Here's how the part is built. I have some questions about the finished solid (model axes, mm). A direction names the side the tool comes from. Give positions to 0.01 mm unless a question says otherwise; leave off trailing zeros. Loops run counter-clockwise (first coordinate to the right, second up) from the corner with the lowest first, then second, coordinate; pieces in that order, holes last. Notation, with made-up numbers: M 34.25,49 L 93.25,49 A25 cw 93.25,84 Z; hole C 56.25,0.5 d3. An arc over 180 degrees is marked long. Write item = value, one per line. Start each with the question number.
```python
from build123d import *

# Parameters (mm, degrees)
SKETCH_1_R      = 41.5
EXTRUDE_1_DEPTH = 2


with BuildPart() as part:
    # 草图1 → 凸台-拉伸1 (new body)
    with BuildSketch(Plane.XY):
        with BuildLine():
            Line((3, -140.066053532), (3, -45.918827896))
            ThreePointArc((3, -45.918827896), (31.460201745, 33.582651198), (-46.016722562, 0))
            Line((-46.016722562, 0), (-46.016722562, -112.361648418))
            ThreePointArc((-46.016722562, -112.361648418), (-37.365245186, -155.855562297), (-12.727922061, -192.727922061))
            ThreePointArc((-12.727922061, -192.727922061), (12.295990665, -193.145669004), (13.548765941, -168.149643825))
            ThreePointArc((13.548765941, -168.149643825), (5.724176996, -155.065757751), (3, -140.066053532))
        make_face()
        Circle(SKETCH_1_R, mode=Mode.SUBTRACT)
    extrude(amount=EXTRUDE_1_DEPTH)


solid = part.part
```
Q1. Will these pins go through, and if not, where does the flat tip stop? pin 1 (1 mm diameter, centred on y = -106, z = 1, fed in from +X); pin 2 (1 mm diameter, centred on x = 26, z = 1, fed in from +Y).
Q2. If we section it at B-B, the plane x = 0: List the corners of the cut face in (y, z) for me.
Q3. If we section it at D-D, the plane x = -10.5: List the corners of the cut face in (y, z) for me, then the cut area to 3 significant figures.
Q4. If we section it at C-C, the plane y = -104: List the corners of the cut face in (x, z) for me, then the cut area to 3 significant figures.
Q5. If I drill on line 1 along Y through (x, z) = (0, 1.55); line 2 along Y through (x, z) = (12, 0.45); line 3 along X through (y, z) = (-14, 1.85), over which ranges is the centre line in solid material (lowest first)?
Q6. We'd pull the mould along X, two halves only. Please class faces 3 (the cylindrical face through (39.584, 12.465, 0.986)), 4 (the cylindrical face through (-37.6, -155.28, 0.99)), 5 (the cylindrical face through (32.54, 32.54, 0.99)), 6 (the flat face through (-21, -101, 2)): pulls with the +X half, pulls with the -X half, needs draft (parallel to the pull), parting line crosses it, or undercut.
Q7. If we section it at A-A, the plane z = 1.45: List the corners of the cut face in (x, y) for me, then the cut area to 3 significant figures.
Q8. On a 3-axis mill with a long thin cutter (end or side, diameter ignored), from which of +Z, -Z, +X, -X, +Y, -Y can I reach the whole of each face in a straight line? I mean faces 1 (the cylindrical face through (12.01, -193.41, 0.99)), 2 (the cylindrical face through (5.8, -155.27, 0.99)). Say none if no direction works.
Resolved:
q1.pin_1 = 3
q1.pin_2 = 38.31
q2.outline = M -198,0 L -41.5,0 L -41.5,2 L -198,2 Z; M 41.5,0 L 46.02,0 L 46.02,2 L 41.5,2 Z
q3.outline = M -194.62,0 L -40.15,0 L -40.15,2 L -194.62,2 Z; M 40.15,0 L 44.8,0 L 44.8,2 L 40.15,2 Z
q3.area = 318 mm²
q4.outline = M -46.02,0 L 3,0 L 3,2 L -46.02,2 Z
q4.area = 98.0 mm²
q5.line_1 = -198 to -41.5, 41.5 to 46.02
q5.line_2 = -193.42 to -166.27, -44.42 to -39.73, 39.73 to 44.42
q5.line_3 = -46.02 to -39.07, 39.07 to 43.84
q6.face_3 = undercut
q6.face_4 = pulls with the -X half
q6.face_5 = parting line crosses it
q6.face_6 = needs draft
q7.outline = M -46.02,-112.36 A113.66 ccw -12.73,-192.73 A18 ccw 13.55,-168.15 A42.66 cw 3,-140.07 L 3,-45.92 A46.02 ccw long -46.02,0 Z; hole C 0,0 d83
q7.area = 8,570 mm²
q8.face_1 = +Z, -Z
q8.face_2 = +Z, -Z, +X
